from build123d import *

# Parameters (mm, degrees)
SKETCH1_W           = 25
SKETCH1_H           = 25
SKETCH1_R           = 0.7
BOSS_EXTRUDE2_DEPTH = 1


with BuildPart() as part:
    # Sketch1 → Boss-Extrude2 (new body)
    with BuildSketch(Plane(origin=(0, 0, 0), x_dir=(1, 0, 0), z_dir=(0, 1, 0))):
        Rectangle(SKETCH1_W, SKETCH1_H)
        with Locations((-8.39, 8.51)):
            Circle(SKETCH1_R, mode=Mode.SUBTRACT)
        with Locations((-6.04, 8.51)):
            Circle(SKETCH1_R, mode=Mode.SUBTRACT)
        with Locations((-3.69, 8.51)):
            Circle(SKETCH1_R, mode=Mode.SUBTRACT)
        with Locations((3.36, 8.51)):
            Circle(SKETCH1_R, mode=Mode.SUBTRACT)
        with Locations((5.71, 8.51)):
            Circle(SKETCH1_R, mode=Mode.SUBTRACT)
        with Locations((8.06, 8.51)):
            Circle(SKETCH1_R, mode=Mode.SUBTRACT)
        with Locations((-6.04, 6.16)):
            Circle(SKETCH1_R, mode=Mode.SUBTRACT)
        with Locations((-3.69, 6.16)):
            Circle(SKETCH1_R, mode=Mode.SUBTRACT)
        with Locations((3.36, 6.16)):
            Circle(SKETCH1_R, mode=Mode.SUBTRACT)
        with Locations((5.71, 6.16)):
            Circle(SKETCH1_R, mode=Mode.SUBTRACT)
        with Locations((8.06, 6.16)):
            Circle(SKETCH1_R, mode=Mode.SUBTRACT)
        with Locations((-6.04, 3.81)):
            Circle(SKETCH1_R, mode=Mode.SUBTRACT)
        with Locations((-3.69, 3.81)):
            Circle(SKETCH1_R, mode=Mode.SUBTRACT)
        with Locations((3.36, 3.81)):
            Circle(SKETCH1_R, mode=Mode.SUBTRACT)
        with Locations((5.71, 3.81)):
            Circle(SKETCH1_R, mode=Mode.SUBTRACT)
        with Locations((8.06, 3.81)):
            Circle(SKETCH1_R, mode=Mode.SUBTRACT)
        with Locations((-8.39, 6.16)):
            Circle(SKETCH1_R, mode=Mode.SUBTRACT)
        with Locations((-8.39, 3.81)):
            Circle(SKETCH1_R, mode=Mode.SUBTRACT)
        with Locations((-6.04, -3.24)):
            Circle(SKETCH1_R, mode=Mode.SUBTRACT)
        with Locations((-3.69, -3.24)):
            Circle(SKETCH1_R, mode=Mode.SUBTRACT)
        with Locations((3.36, -3.24)):
            Circle(SKETCH1_R, mode=Mode.SUBTRACT)
        with Locations((5.71, -3.24)):
            Circle(SKETCH1_R, mode=Mode.SUBTRACT)
        with Locations((8.06, -3.24)):
            Circle(SKETCH1_R, mode=Mode.SUBTRACT)
        with Locations((-6.04, -5.59)):
            Circle(SKETCH1_R, mode=Mode.SUBTRACT)
        with Locations((-3.69, -5.59)):
            Circle(SKETCH1_R, mode=Mode.SUBTRACT)
        with Locations((3.36, -5.59)):
            Circle(SKETCH1_R, mode=Mode.SUBTRACT)
        with Locations((5.71, -5.59)):
            Circle(SKETCH1_R, mode=Mode.SUBTRACT)
        with Locations((8.06, -5.59)):
            Circle(SKETCH1_R, mode=Mode.SUBTRACT)
        with Locations((-6.04, -7.94)):
            Circle(SKETCH1_R, mode=Mode.SUBTRACT)
        with Locations((-3.69, -7.94)):
            Circle(SKETCH1_R, mode=Mode.SUBTRACT)
        with Locations((3.36, -7.94)):
            Circle(SKETCH1_R, mode=Mode.SUBTRACT)
        with Locations((5.71, -7.94)):
            Circle(SKETCH1_R, mode=Mode.SUBTRACT)
        with Locations((8.06, -7.94)):
            Circle(SKETCH1_R, mode=Mode.SUBTRACT)
        with Locations((-8.39, -3.24)):
            Circle(SKETCH1_R, mode=Mode.SUBTRACT)
        with Locations((-8.39, -5.59)):
            Circle(SKETCH1_R, mode=Mode.SUBTRACT)
        with Locations((-8.39, -7.94)):
            Circle(SKETCH1_R, mode=Mode.SUBTRACT)
    extrude(amount=BOSS_EXTRUDE2_DEPTH)


solid = part.part
Work out the finished part from the listing and answer in its coordinate system (mm). Give positions to 0.01 mm unless a question says otherwise; leave off trailing zeros. Write each loop counter-clockwise with the first axis right and the second up, starting at its lowest first coordinate (ties: lowest second). Pieces come first, ordered by that corner, then holes. Notation, with made-up numbers: (84.25, -7.75) - (102.25, -7.75) arc R14 ccw to (102.25, 16.25) - close; hole circle Ø2 at (73.5, 23). An arc over 180 degrees is marked (long way). One line per item, written item: value. Start each with the question number.
1. Given pin 1 (1.1 mm diameter, centred on x = -3.69, z = -3.81, fed in from -Y), flat-ended and moving along its own axis, determine where the tip first touches the part or whether it passes through.
2. Find section A-A (x = 5.71). Write down the section's boundary in (y, z).
3. Find section C-C (y = 0.85). State how many separate pieces and enclosed holes the cut face has, then the cut area to 3 significant figures.
4. For a pull along X with two mould halves and no side action, classify faces 1 (the flat face through (-0.2, 0.5, 12.5)), 2 (the cylindrical face through (7.505, 0.493, -5.734)), 3 (the cylindrical face through (7.54, 0.49, 7.47)) as +X half, -X half, draft (parallel to the pull), parting line (faces both ways), or undercut.
5. Find section B-B (z = 7.94). Write down the section's boundary in (x, y).
Geometry results:
1. pin 1: through
2. outline: (0, -12.5) - (1, -12.5) - (1, -9.21) - (0, -9.21) - close; (0, -7.81) - (1, -7.81) - (1, -6.86) - (0, -6.86) - close; (0, -5.46) - (1, -5.46) - (1, -4.51) - (0, -4.51) - close; (0, -3.11) - (1, -3.11) - (1, 2.54) - (0, 2.54) - close; (0, 3.94) - (1, 3.94) - (1, 4.89) - (0, 4.89) - close; (0, 6.29) - (1, 6.29) - (1, 7.24) - (0, 7.24) - close; (0, 8.64) - (1, 8.64) - (1, 12.5) - (0, 12.5) - close
3. separate pieces: 1
3. enclosed holes: 36
3. area: 570 mm2
4. face 1: draft
4. face 2: undercut
4. face 3: undercut
5. outline: (-12.5, 0) - (-9.09, 0) - (-9.09, 1) - (-12.5, 1) - close; (-7.69, 0) - (-6.74, 0) - (-6.74, 1) - (-7.69, 1) - close; (-5.34, 0) - (-4.39, 0) - (-4.39, 1) - (-5.34, 1) - close; (-2.99, 0) - (2.66, 0) - (2.66, 1) - (-2.99, 1) - close; (4.06, 0) - (5.01, 0) - (5.01, 1) - (4.06, 1) - close; (6.41, 0) - (7.36, 0) - (7.36, 1) - (6.41, 1) - close; (8.76, 0) - (12.5, 0) - (12.5, 1) - (8.76, 1) - close
